Check sheet for the modelled part. Datum: model origin and axes. Units: mm. A direction names the side the tool comes from. Round coordinates to 2 decimals unless told otherwise and drop trailing zeros. Write each loop counter-clockwise with the first axis right and the second up, starting at its lowest first coordinate (ties: lowest second). Pieces come first, ordered by that corner, then holes. Notation, with made-up numbers: (25, 9.5) -> (40, 9.5) arc R32 ccw to (40, 46.5) -> close; hole circle Ø4 at (75, -23). An arc over 180 degrees is marked (long way). Use one line per item in the form item = value. Start each with the question number.
```python
from build123d import *

# Parameters (mm, degrees)
BOSS_EXTRUDE1_DEPTH = 24
BOSS_EXTRUDE2_START = 47
SKETCH2_W           = 80
SKETCH2_H           = 24
BOSS_EXTRUDE2_DEPTH = 36


with BuildPart() as part:
    # Sketch1 → Boss-Extrude1 (new, symmetric)
    with BuildSketch(Plane.XY):
        Polygon((-14, 10.891224152), (0, 10.891224152), (0, 38), (-21, 38), (-46, 13), (-46, 0), (-14, 0), align=None)
        Polygon((14, 10.891224152), (14, 0), (46, 0), (46, 13), (21, 38), (0, 38), (0, 10.891224152), align=None)
    extrude(amount=BOSS_EXTRUDE1_DEPTH, both=True)

    # Sketch2 → Boss-Extrude2 (add)
    with BuildSketch(Plane(origin=(0, 0, 0), x_dir=(1, 0, 0), z_dir=(0, 1, 0)).offset(BOSS_EXTRUDE2_START)):
        Rectangle(SKETCH2_W, SKETCH2_H)
    extrude(amount=-BOSS_EXTRUDE2_DEPTH)


solid = part.part
```
1. Sectioned sample at D-D (y = 28). Enter the section's corners in (x, z), and give its area (3 significant figures).
2. Depth check by flat-ended pin: pin 1 (2 mm diameter, centred on x = -12, z = -4, fed in from -Y); pin 2 (7 mm diameter, centred on y = 31, z = -1.5, fed in from +X); pin 3 (6 mm diameter, centred on x = -10.5, z = 19.5, fed in from +Y); pin 4 (3 mm diameter, centred on y = 13.5, z = -3.5, fed in from -X). Enter the tip coordinate at first touch or a pass-through.
3. Sectioned sample at C-C (x = -16). Enter the section's corners in (y, z), and give its area (3 significant figures).
4. Mould release check, pull along X, two halves, no side actions. Record for faces 1 (the face through (-40, 33, 0)), 2 (the face through (0, 10.891, 0)), 3 (the face through (14, 6, 0)), 4 (the face through (-1, 19, 24)): +X half, -X half, draft (parallel to the pull), parting line (faces both ways), or undercut.
5. Sectioned sample at A-A (y = 5.5). Enter the section's corners in (x, z).
6. Scan lines: probe 1 along X at (y, z) = (3.5, 12); probe 2 along X at (y, z) = (24, 1.5); probe 3 along Y at (x, z) = (-1.5, 5). Record each from-to range of solid material in increasing order.
7. Tool access check on faces 5 (the face through (40, 33, 0)), 6 (the face through (-1, 39, -12)), 7 (the face through (-1, 39, 12)), 8 (the face through (0, 38, 18)). Record the directions out of +Z, -Z, +X, -X, +Y, -Y that give a thin tool (end or side, any length) a straight path to the whole face; none if there is none.
8. Sectioned sample at B-B (z = 18.5). Enter the section's corners in (x, y), and give its area (3 significant figures).
Returned:
q1.outline = (-40, -12) -> (-31, -12) -> (-31, -24) -> (31, -24) -> (31, -12) -> (40, -12) -> (40, 12) -> (31, 12) -> (31, 24) -> (-31, 24) -> (-31, 12) -> (-40, 12) -> close
q1.area = 3,410 mm^2
q2.pin_1 = 10.89
q2.pin_2 = 40
q2.pin_3 = 38
q2.pin_4 = -46
q3.outline = (0, -24) -> (38, -24) -> (38, -12) -> (47, -12) -> (47, 12) -> (38, 12) -> (38, 24) -> (0, 24) -> close
q3.area = 2,040 mm^2
q4.face_1 = -X half
q4.face_2 = undercut
q4.face_3 = undercut
q4.face_4 = draft
q5.outline = (-46, -24) -> (-14, -24) -> (-14, 24) -> (-46, 24) -> close; (14, -24) -> (46, -24) -> (46, 24) -> (14, 24) -> close
q6.probe_1 = -46 to -14, 14 to 46
q6.probe_2 = -40 to 40
q6.probe_3 = 10.89 to 47
q7.face_5 = +Z, -Z, +X, +Y
q7.face_6 = -Z, +Y
q7.face_7 = +Z, +Y
q7.face_8 = +Z, +X, -X, +Y
q8.outline = (-46, 0) -> (-14, 0) -> (-14, 10.89) -> (14, 10.89) -> (14, 0) -> (46, 0) -> (46, 13) -> (21, 38) -> (-21, 38) -> (-46, 13) -> close
q8.area = 2,570 mm^2
